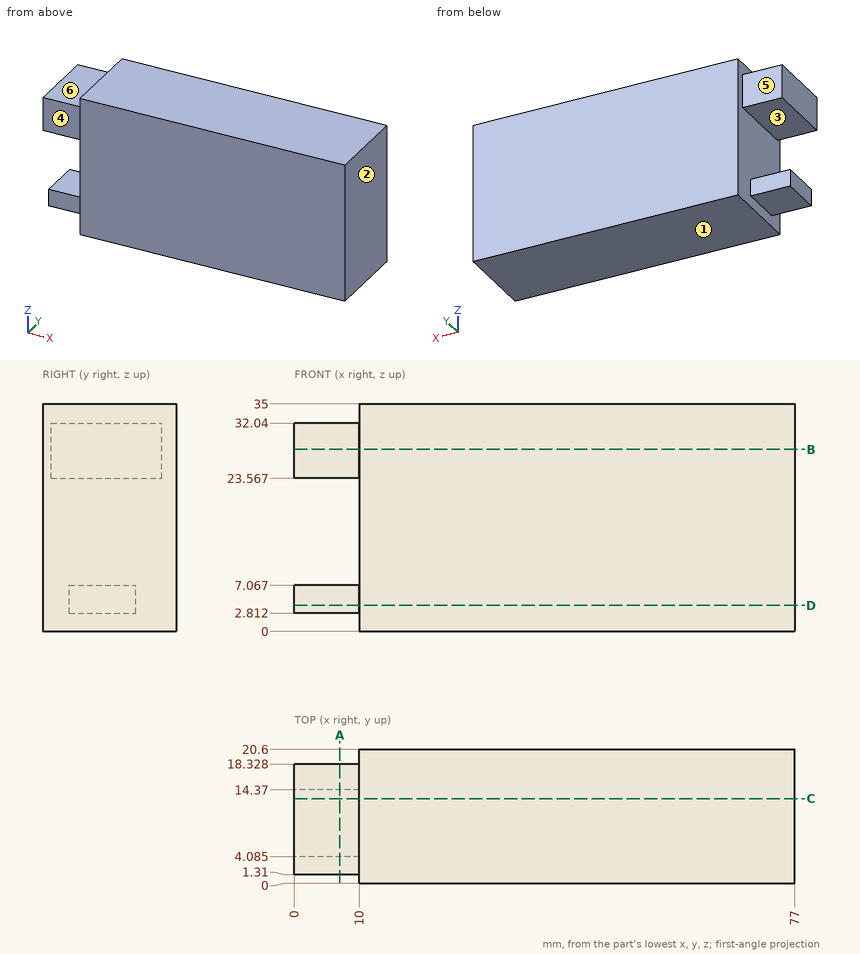
The drawing under review shows one solid part. Ordinate dimensions are in mm from its lowest x, y, z. A direction names the side the tool comes from. Coordinates: 2 decimals unless noted, no trailing zeros. Write each loop counter-clockwise with the first axis right and the second up, starting at its lowest first coordinate (ties: lowest second). Pieces come first, ordered by that corner, then holes. Notation, with made-up numbers: (7.5, 83) - (47.5, 83) arc R27 ccw to (47.5, 100) - close; hole circle Ø6 at (89.5, 72.25). An arc over 180 degrees is marked (long way). Answer as CSV lines item,"result".
(1) For line 1 along Z through (x, y) = (4, 12); line 2 along X through (y, z) = (19, 11.5); line 3 along Z through (x, y) = (6, 2.5), list the stretches that pass through material, from the lowest coordinate up. Write a range as [from, to].
Data:
line 1,"z = [2.81, 7.07], [23.57, 32.04]"
line 2,"x = [10, 77]"
line 3,"z = [23.57, 32.04]"
(2) Clearance check with flat-ended pins moving along their axes: pin 1 Ø4 at (y, z) = (14, 23) entering from -X; pin 2 Ø4.5 at (x, z) = (3, 5) entering from -Y (1 decimal); pin 3 Ø8 at (x, y) = (4.5, 13) entering from -Z; pin 4 Ø4 at (x, z) = (5.5, 28) entering from +Y. State where each tip first meets the part, or that it passes through.
Data:
pin 1,"stops at x = 0"
pin 2,"stops at y = 4.1"
pin 3,"stops at z = 2.81"
pin 4,"stops at y = 18.33"
(3) We need section A-A (x = 7). Give the boundary of the cut face in (y, z) (1 decimal).
Data:
outline,"(1.3, 23.6) - (18.3, 23.6) - (18.3, 32) - (1.3, 32) - close; (4.1, 2.8) - (14.4, 2.8) - (14.4, 7.1) - (4.1, 7.1) - close"
(4) Mouldability with a two-part tool opening along Z and no side actions: class the marked faces 1, 2 and 3 as pulls with the +Z half, pulls with the -Z half, needs draft (parallel to the pull), parting line crosses it, or undercut.
Data:
face 1,"pulls with the -Z half"
face 2,"needs draft"
face 3,"undercut"
(5) We need section D-D (z = 4). Give the boundary of the cut face in (x, y) (1 decimal), plus the area to 3 significant figures.
Data:
outline,"(0, 4.1) - (10, 4.1) - (10, 0) - (77, 0) - (77, 20.6) - (10, 20.6) - (10, 14.4) - (0, 14.4) - close"
area,"1,480 mm2"
(6) We need section B-B (z = 28). Give the boundary of the cut face in (x, y).
Data:
outline,"(0, 1.31) - (10, 1.31) - (10, 0) - (77, 0) - (77, 20.6) - (10, 20.6) - (10, 18.33) - (0, 18.33) - close"
(7) Tool access review of the marked faces 4, 5 and 6: name each direction out of +Z, -Z, +X, -X, +Y, -Y from which nothing blocks a thin tool from reaching the whole face with its end or side.
Data:
face 4,"+Z, -Z, -X, -Y"
face 5,"+Z, -Z, -X, +Y"
face 6,"+Z, -X, +Y, -Y"
(8) We need section C-C (y = 13). Give the boundary of the cut face in (x, z), plus the area to 3 significant figures.
Data:
outline,"(0, 2.81) - (10, 2.81) - (10, 0) - (77, 0) - (77, 35) - (10, 35) - (10, 32.04) - (0, 32.04) - (0, 23.57) - (10, 23.57) - (10, 7.07) - (0, 7.07) - close"
area,"2,470 mm2"
